from build123d import *

# Parameters (mm, degrees)
SKETCH1_W           = 600
SKETCH1_H           = 1800
BOSS_EXTRUDE1_DEPTH = 650
SHELL1_T            = -20
BOSS_EXTRUDE2_REACH = 1152
SKETCH2_W           = 5
SKETCH2_H           = 5


with BuildPart() as part:
    # Sketch1 → Boss-Extrude1 (new body)
    with BuildSketch(Plane.XY):
        Rectangle(SKETCH1_W, SKETCH1_H)
    extrude(amount=BOSS_EXTRUDE1_DEPTH)

    # Shell1
    shell1_openings = [part.faces().sort_by_distance(p)[0] for p in [
        (0, 0, 650),
    ]]
    offset(amount=SHELL1_T, openings=shell1_openings, kind=Kind.INTERSECTION)

    # Sketch2 → Boss-Extrude2 (add, up to next)
    with BuildSketch(Plane.XY.offset(650), mode=Mode.PRIVATE) as boss_extrude2_sk1:
        with Locations((277.5, 521.5)):
            Rectangle(SKETCH2_W, SKETCH2_H)
    boss_extrude2_tool1 = extrude(boss_extrude2_sk1.sketch, amount=-BOSS_EXTRUDE2_REACH, mode=Mode.PRIVATE) - part.part
    # Sketch2 → Boss-Extrude2 (add, up to next)
    with BuildSketch(Plane.XY.offset(650), mode=Mode.PRIVATE) as boss_extrude2_sk2:
        with Locations((277.5, 165.5)):
            Rectangle(SKETCH2_W, SKETCH2_H)
    boss_extrude2_tool2 = extrude(boss_extrude2_sk2.sketch, amount=-BOSS_EXTRUDE2_REACH, mode=Mode.PRIVATE) - part.part
    # Sketch2 → Boss-Extrude2 (add, up to next)
    with BuildSketch(Plane.XY.offset(650), mode=Mode.PRIVATE) as boss_extrude2_sk3:
        with Locations((277.5, -190.5)):
            Rectangle(SKETCH2_W, SKETCH2_H)
    boss_extrude2_tool3 = extrude(boss_extrude2_sk3.sketch, amount=-BOSS_EXTRUDE2_REACH, mode=Mode.PRIVATE) - part.part
    # Sketch2 → Boss-Extrude2 (add, up to next)
    with BuildSketch(Plane.XY.offset(650), mode=Mode.PRIVATE) as boss_extrude2_sk4:
        with Locations((277.5, -546.5)):
            Rectangle(SKETCH2_W, SKETCH2_H)
    boss_extrude2_tool4 = extrude(boss_extrude2_sk4.sketch, amount=-BOSS_EXTRUDE2_REACH, mode=Mode.PRIVATE) - part.part
    boss_extrude2_1 = boss_extrude2_tool1.solids().sort_by_distance((277.5, 521.5, 650))[0]
    add(boss_extrude2_1)
    boss_extrude2_2 = boss_extrude2_tool2.solids().sort_by_distance((277.5, 165.5, 650))[0]
    add(boss_extrude2_2)
    boss_extrude2_3 = boss_extrude2_tool3.solids().sort_by_distance((277.5, -190.5, 650))[0]
    add(boss_extrude2_3)
    boss_extrude2_4 = boss_extrude2_tool4.solids().sort_by_distance((277.5, -546.5, 650))[0]
    add(boss_extrude2_4)
    boss_extrude2 = boss_extrude2_1 + boss_extrude2_2 + boss_extrude2_3 + boss_extrude2_4  # Boss-Extrude2 as one shape, for the pattern or mirror that repeats it

    # Mirror1: Boss-Extrude2 across plane
    add(boss_extrude2.mirror(Plane(origin=(0, 0, 0), x_dir=(0, 0, 1), z_dir=(1, 0, 0))))


solid = part.part
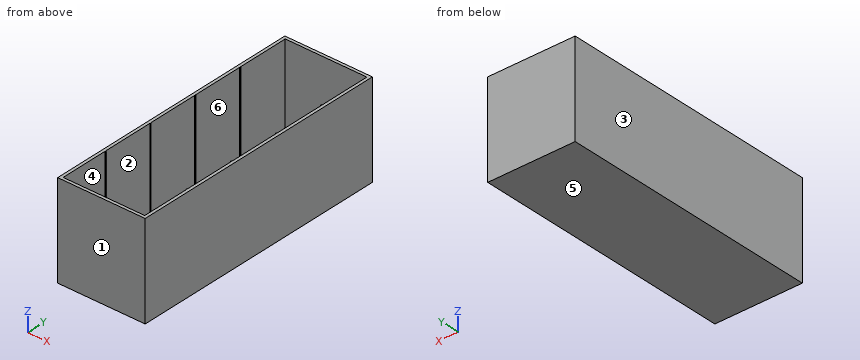
Geometry: final body of the model. Coordinates: model frame, mm. Face numbers are marked on the shaded views. A direction names the side the tool comes from. Coordinates: 2 decimals unless noted, no trailing zeros. Order: outer loops, then holes, each group sorted by start corner. A loop starts at its lowest first (then second) coordinate and runs counter-clockwise, first axis right, second up.
(1) Section query B-B (y = 406.5). Return the cut outline in (x, z), plus the area to 3 significant figures.
(2) Section query A-A (x = -152). Return the cut outline in (y, z), plus the area to 3 significant figures.
(3) Draft query along X for the marked faces 1, 2, 3 and 4. Return one class per face: pulls with the +X half, pulls with the -X half, needs draft (parallel to the pull), parting line crosses it, or undercut.
(4) First-contact query: pin 1 (6 mm diameter, centred on x = 99, y = -74, fed in from +Z). Flat tip, straight axial feed; report the tip coordinate or a pass-through.
(5) Access query for the marked faces 5 and 6. Directions: +Z, -Z, +X, -X, +Y, -Y. A direction counts if a zero-diameter tool reaches every point of the face in a straight line with its end or side. Return the directions, or none.
(6) Material intervals for probe 1 along X at (y, z) = (457, 200.5); probe 2 along Y at (x, z) = (19.5, 565); probe 3 along Z at (x, y) = (28, 511.5), sorted ascending.
Solution:
1. outline: (-300, 0) - (300, 0) - (300, 650) - (280, 650) - (280, 20) - (-280, 20) - (-280, 650) - (-300, 650) - close
1. area: 37,200 mm2
2. outline: (-900, 0) - (900, 0) - (900, 650) - (880, 650) - (880, 20) - (-880, 20) - (-880, 650) - (-900, 650) - close
2. area: 61,200 mm2
3. face 1: needs draft
3. face 2: undercut
3. face 3: pulls with the -X half
3. face 4: undercut
4. pin 1: stops at z = 20
5. face 5: -Z, +X, -X, +Y, -Y
5. face 6: +Z
6. probe 1: x = -300 to -280, 280 to 300
6. probe 2: y = -900 to -880, 880 to 900
6. probe 3: z = 0 to 20
